from build123d import *

# Parameters (mm, degrees)
F0_R     = 4.25
F1_DEPTH = 250


with BuildPart() as f1:
    # F0 (on Front) → F1 (new body)
    with BuildSketch(Plane.XZ):
        Polygon((-4.5, -5), (4.5, -5), (5, -5), (5, -4.5), (5, 4.5), (5, 5), (4.5, 5), (-4.5, 5), (-5, 5), (-5, 4.5), (-5, -4.5), (-5, -5), align=None)
        Circle(F0_R, mode=Mode.SUBTRACT)
    extrude(amount=F1_DEPTH)


solid = f1.part
Geometry: final body of the model. Coordinates: model frame, mm. Give positions to 0.01 mm unless a question says otherwise; leave off trailing zeros. Write each loop counter-clockwise with the first axis right and the second up, starting at its lowest first coordinate (ties: lowest second). Pieces come first, ordered by that corner, then holes. Notation, with made-up numbers: (76, -29) -> (110, -29) arc R16 cw to (110, -20) -> close; hole circle Ø5 at (65, 4). An arc over 180 degrees is marked (long way). Answer in a Markdown table with one row per item.
(1) Section query A-A on z = 0. Return loops of the section in (x, y), then the cut area to 3 significant figures.
Answers below:
| item | result |
|---|---|
| outline | (-5, -250) -> (-4.25, -250) -> (-4.25, 0) -> (-5, 0) -> close; (4.25, -250) -> (5, -250) -> (5, 0) -> (4.25, 0) -> close |
| area | 375 mm^2 |
(2) Section query C-C on y = -115. Return loops of the section in (x, z), then the cut area to 3 significant figures.
Answers below:
| item | result |
|---|---|
| outline | (-5, -5) -> (5, -5) -> (5, 5) -> (-5, 5) -> close; hole circle Ø8.5 at (0, 0) |
| area | 43.3 mm^2 |
(3) Draft query along Z for faces 1 (the cylindrical face through (2.285, -123.25, 3.584)), 2 (the flat face through (0, -123, -5)), 3 (the flat face through (0, -123, 5)). Return one class per face: +Z half, -Z half, draft (parallel to the pull), parting line (faces both ways), or undercut.
Answers below:
| item | result |
|---|---|
| face 1 | undercut |
| face 2 | -Z half |
| face 3 | +Z half |
(4) Section query B-B on x = 2. Return loops of the section in (y, z), then the cut area to 3 significant figures.
Answers below:
| item | result |
|---|---|
| outline | (-250, -5) -> (0, -5) -> (0, -3.75) -> (-250, -3.75) -> close; (-250, 3.75) -> (0, 3.75) -> (0, 5) -> (-250, 5) -> close |
| area | 625 mm^2 |
(5) Ray query, line 1 along Z through (x, y) = (0, -103); line 2 along Z through (x, y) = (2.5, -237.5); line 3 along X through (y, z) = (-57.5, 2.25). Return the intervals inside material, ascending. Write a range as [from, to].
Answers below:
| item | result |
|---|---|
| line 1 | [-5, -4.25], [4.25, 5] |
| line 2 | [-5, -3.44], [3.44, 5] |
| line 3 | [-5, -3.61], [3.61, 5] |
